from build123d import *

# Parameters (mm, degrees)
F0_R     = 1.5
F0_R_2   = 3.5
F0_R_3   = 1
F0_R_4   = 2.0426148112
F1_DEPTH = 4


with BuildPart() as f1:
    # F0 (on Top) → F1 (new body)
    with BuildSketch(Plane.XY):
        with BuildLine():
            Line((28.2485083335, 43.9163537211), (28.2485083335, 54.5580207216))
            ThreePointArc((28.2485083335, 54.5580207216), (27.1525007025, 57.2380411405), (24.4926270097, 58.38207528))
            Line((24.4926270097, 58.38207528), (15.9756345674, 58.38207528))
            ThreePointArc((15.9756345674, 58.38207528), (11.5015417116, 56.5288453398), (9.6483117715, 52.054752484))
            Line((9.6483117715, 52.054752484), (9.6483117715, 39.0478140861))
            ThreePointArc((9.6483117715, 39.0478140861), (7.7950818313, 34.5737212303), (3.3209889755, 32.7204912901))
            Line((3.3209889755, 32.7204912901), (0, 32.7204912901))
            Line((0, 32.7204912901), (-3.3209889755, 32.7204912901))
            ThreePointArc((-3.3209889755, 32.7204912901), (-7.7950818313, 34.5737212303), (-9.6483117715, 39.0478140861))
            Line((-9.6483117715, 39.0478140861), (-9.6483117715, 52.054752484))
            ThreePointArc((-9.6483117715, 52.054752484), (-11.5015417116, 56.5288453398), (-15.9756345674, 58.38207528))
            Line((-15.9756345674, 58.38207528), (-24.4926270097, 58.38207528))
            ThreePointArc((-24.4926270097, 58.38207528), (-27.1525007025, 57.2380411405), (-28.2485083335, 54.5580207216))
            Line((-28.2485083335, 54.5580207216), (-28.2485083335, 43.9163537211))
            ThreePointArc((-28.2485083335, 43.9163537211), (-30.8923065557, 39.5063295508), (-36.0278336063, 39.759991005))
            Line((-36.0278336063, 39.759991005), (-83.3553595539, 71.4075150422))
            ThreePointArc((-83.3553595539, 71.4075150422), (-83.1773407039, 70.0948228733), (-83.1178410423, 68.7714517117))
            ThreePointArc((-83.1178410423, 68.7714517117), (-86.7609350808, 59.0670533301), (-95.8902072963, 54.1574840073))
            Line((-95.8902072963, 54.1574840073), (-30.0196265199, 1.5012365572))
            ThreePointArc((-30.0196265199, 1.5012365572), (-28.6355347687, -0.2374876701), (-28.1416475773, -2.4042703903))
            Line((-28.1416475773, -2.4042703903), (-28.1416475773, -40))
            ThreePointArc((-28.1416475773, -40), (-28.0556598352, -40.8267401557), (-27.8013775488, -41.6180894438))
            Line((-27.8013775488, -41.6180894438), (-21.7254169173, -55.4257667582))
            ThreePointArc((-21.7254169173, -55.4257667582), (-21.5878462389, -55.7131878969), (-21.4322469923, -55.9912624857))
            Line((-21.4322469923, -55.9912624857), (-10.7166659506, -73.7858242134))
            ThreePointArc((-10.7166659506, -73.7858242134), (-10.1824970033, -75.0266439297), (-10, -76.3651747946))
            Line((-10, -76.3651747946), (-10, -176.3651747946))
            Line((-10, -176.3651747946), (-17.5625588745, -176.3651747946))
            Line((-17.5625588745, -176.3651747946), (-17.5625588745, -183.6033910513))
            Line((-17.5625588745, -183.6033910513), (0, -183.6033910513))
            Line((0, -183.6033910513), (17.5625588745, -183.6033910513))
            Line((17.5625588745, -183.6033910513), (17.5625588745, -176.3651747946))
            Line((17.5625588745, -176.3651747946), (10, -176.3651747946))
            Line((10, -176.3651747946), (10, -76.3651747946))
            ThreePointArc((10, -76.3651747946), (10.1824970033, -75.0266439297), (10.7166659506, -73.7858242134))
            Line((10.7166659506, -73.7858242134), (21.4322469923, -55.9912624857))
            ThreePointArc((21.4322469923, -55.9912624857), (21.5878462389, -55.7131878969), (21.7254169173, -55.4257667582))
            Line((21.7254169173, -55.4257667582), (27.8013775488, -41.6180894438))
            ThreePointArc((27.8013775488, -41.6180894438), (28.0556598352, -40.8267401557), (28.1416475773, -40))
            Line((28.1416475773, -40), (28.1416475773, -2.4042703903))
            ThreePointArc((28.1416475773, -2.4042703903), (28.6355347687, -0.2374876701), (30.0196265199, 1.5012365572))
            Line((30.0196265199, 1.5012365572), (95.8902072963, 54.1574840073))
            ThreePointArc((95.8902072963, 54.1574840073), (85.9348635201, 60.1026484333), (83.3553595539, 71.4075150422))
            Line((83.3553595539, 71.4075150422), (36.0278336063, 39.759991005))
            ThreePointArc((36.0278336063, 39.759991005), (30.8923065557, 39.5063295508), (28.2485083335, 43.9163537211))
        make_face()
        with BuildLine():
            ThreePointArc((0, -96.7485921342), (1.1190603643, -97.1534205019), (1.5911210664, -98.2458218932))
            ThreePointArc((1.5911210664, -98.2458218932), (1.1190603643, -99.3382232845), (0, -99.7430516522))
            ThreePointArc((0, -99.7430516522), (-1.5911210664, -98.2458218932), (0, -96.7485921342))
        make_face(mode=Mode.SUBTRACT)
        with Locations((-15, -44.9954515789)):
            Circle(F0_R, mode=Mode.SUBTRACT)
        with Locations((-66.8339952826, 46.3828593493)):
            Circle(F0_R, mode=Mode.SUBTRACT)
        with Locations((-29.9585536122, 18.5773223639)):
            Circle(F0_R, mode=Mode.SUBTRACT)
        with Locations((-18.9252551645, 47.9994341731)):
            Circle(F0_R, mode=Mode.SUBTRACT)
        with Locations((0, -44.9723601341)):
            Circle(F0_R_2, mode=Mode.SUBTRACT)
        with Locations((15, -44.9954515789)):
            Circle(F0_R, mode=Mode.SUBTRACT)
        with BuildLine():
            ThreePointArc((-10.1997302845, 5.3493127972), (-8.7352641904, 8.8848467031), (-5.1997302845, 10.3493127972))
            Line((-5.1997302845, 10.3493127972), (5.4373050854, 10.3493127972))
            ThreePointArc((5.4373050854, 10.3493127972), (8.9728389913, 8.8848467031), (10.4373050854, 5.3493127972))
            Line((10.4373050854, 5.3493127972), (10.4373050854, -5.1066948846))
            ThreePointArc((10.4373050854, -5.1066948846), (8.9728389913, -8.6422287905), (5.4373050854, -10.1066948846))
            Line((5.4373050854, -10.1066948846), (-5.1997302845, -10.1066948846))
            ThreePointArc((-5.1997302845, -10.1066948846), (-8.7352641904, -8.6422287905), (-10.1997302845, -5.1066948846))
            Line((-10.1997302845, -5.1066948846), (-10.1997302845, 5.3493127972))
        make_face(mode=Mode.SUBTRACT)
        with Locations((18.9252551645, 47.9994341731)):
            Circle(F0_R, mode=Mode.SUBTRACT)
        with Locations((29.9585536122, 18.5773223639)):
            Circle(F0_R, mode=Mode.SUBTRACT)
        with Locations((66.8339952826, 46.3828593493)):
            Circle(F0_R, mode=Mode.SUBTRACT)
        with BuildLine():
            ThreePointArc((112.4534682434, 70.9232873205), (98.1099452114, 83.5161448719), (83.3553595539, 71.4075150422))
            Line((83.3553595539, 71.4075150422), (98.6924420624, 81.6632949003))
            ThreePointArc((98.6924420624, 81.6632949003), (102.2363175022, 82.4481327511), (105.3772742827, 80.6289532416))
            Line((105.3772742827, 80.6289532416), (111.4671739885, 73.0107645192))
            ThreePointArc((111.4671739885, 73.0107645192), (112.0824576726, 72.0247331774), (112.4534682434, 70.9232873205))
        make_face()
        with BuildLine():
            Line((98.6924420624, 81.6632949003), (83.3553595539, 71.4075150422))
            ThreePointArc((83.3553595539, 71.4075150422), (85.9348635201, 60.1026484333), (95.8902072963, 54.1574840073))
            Line((95.8902072963, 54.1574840073), (110.6836880983, 65.9832365143))
            ThreePointArc((110.6836880983, 65.9832365143), (112.0902955562, 67.7694219265), (112.5605632629, 69.9937985024))
            ThreePointArc((112.5605632629, 69.9937985024), (112.514389285, 70.4593924844), (112.4534682434, 70.9232873205))
            ThreePointArc((112.4534682434, 70.9232873205), (112.0824576726, 72.0247331774), (111.4671739885, 73.0107645192))
            Line((111.4671739885, 73.0107645192), (105.3772742827, 80.6289532416))
            ThreePointArc((105.3772742827, 80.6289532416), (102.2363175022, 82.4481327511), (98.6924420624, 81.6632949003))
        make_face()
        with Locations((97.8645756841, 60.7714517117)):
            Circle(F0_R_3, mode=Mode.SUBTRACT)
        with Locations((88.3645756841, 68.7714517117)):
            Circle(F0_R_3, mode=Mode.SUBTRACT)
        with Locations((97.8645756841, 68.7714517117)):
            Circle(F0_R_4, mode=Mode.SUBTRACT)
        with Locations((97.8645756841, 76.7714517117)):
            Circle(F0_R_3, mode=Mode.SUBTRACT)
        with Locations((107.3645756841, 68.7714517117)):
            Circle(F0_R_3, mode=Mode.SUBTRACT)
        with BuildLine():
            ThreePointArc((112.5605632629, 69.9937985024), (112.5288051758, 70.4610534728), (112.4534682434, 70.9232873205))
            ThreePointArc((112.4534682434, 70.9232873205), (112.514389285, 70.4593924844), (112.5605632629, 69.9937985024))
        make_face()
        with BuildLine():
            Line((110.6836880983, 65.9832365143), (95.8902072963, 54.1574840073))
            ThreePointArc((95.8902072963, 54.1574840073), (107.5689740656, 57.6678111084), (112.6113103258, 68.7714517117))
            ThreePointArc((112.6113103258, 68.7714517117), (112.5986180981, 69.3831515852), (112.5605632629, 69.9937985024))
            ThreePointArc((112.5605632629, 69.9937985024), (112.0902955562, 67.7694219265), (110.6836880983, 65.9832365143))
        make_face()
        with BuildLine():
            ThreePointArc((-83.1178410423, 68.7714517117), (-83.1773407039, 70.0948228733), (-83.3553595539, 71.4075150422))
            Line((-83.3553595539, 71.4075150422), (-98.6924420624, 81.6632949003))
            ThreePointArc((-98.6924420624, 81.6632949003), (-102.2363175022, 82.4481327511), (-105.3772742827, 80.6289532416))
            Line((-105.3772742827, 80.6289532416), (-111.4671739885, 73.0107645192))
            ThreePointArc((-111.4671739885, 73.0107645192), (-112.0824576726, 72.0247331774), (-112.4534682434, 70.9232873205))
            ThreePointArc((-112.4534682434, 70.9232873205), (-112.514389285, 70.4593924844), (-112.5605632629, 69.9937985024))
            ThreePointArc((-112.5605632629, 69.9937985024), (-112.0902955562, 67.7694219265), (-110.6836880983, 65.9832365143))
            Line((-110.6836880983, 65.9832365143), (-95.8902072963, 54.1574840073))
            ThreePointArc((-95.8902072963, 54.1574840073), (-86.7609350808, 59.0670533301), (-83.1178410423, 68.7714517117))
        make_face()
        with Locations((-97.8645756841, 60.7714517117)):
            Circle(F0_R_3, mode=Mode.SUBTRACT)
        with Locations((-107.3645756841, 68.7714517117)):
            Circle(F0_R_3, mode=Mode.SUBTRACT)
        with Locations((-97.8645756841, 68.7714517117)):
            Circle(F0_R_4, mode=Mode.SUBTRACT)
        with Locations((-88.3645756841, 68.7714517117)):
            Circle(F0_R_3, mode=Mode.SUBTRACT)
        with Locations((-97.8645756841, 76.7714517117)):
            Circle(F0_R_3, mode=Mode.SUBTRACT)
        with BuildLine():
            Line((-98.6924420624, 81.6632949003), (-83.3553595539, 71.4075150422))
            ThreePointArc((-83.3553595539, 71.4075150422), (-98.1099452114, 83.5161448719), (-112.4534682434, 70.9232873205))
            ThreePointArc((-112.4534682434, 70.9232873205), (-112.0824576726, 72.0247331774), (-111.4671739885, 73.0107645192))
            Line((-111.4671739885, 73.0107645192), (-105.3772742827, 80.6289532416))
            ThreePointArc((-105.3772742827, 80.6289532416), (-102.2363175022, 82.4481327511), (-98.6924420624, 81.6632949003))
        make_face()
        with BuildLine():
            ThreePointArc((-112.5605632629, 69.9937985024), (-112.514389285, 70.4593924844), (-112.4534682434, 70.9232873205))
            ThreePointArc((-112.4534682434, 70.9232873205), (-112.5288051758, 70.4610534728), (-112.5605632629, 69.9937985024))
        make_face()
        with BuildLine():
            ThreePointArc((-112.5605632629, 69.9937985024), (-108.0212046971, 58.0799097421), (-95.8902072963, 54.1574840073))
            Line((-95.8902072963, 54.1574840073), (-110.6836880983, 65.9832365143))
            ThreePointArc((-110.6836880983, 65.9832365143), (-112.0902955562, 67.7694219265), (-112.5605632629, 69.9937985024))
        make_face()
    extrude(amount=F1_DEPTH)


solid = f1.part
Source: CAD feature listing. Evaluate the final solid. Frame: model axes, mm. A direction names the side the tool comes from. Round coordinates to 2 decimals unless told otherwise and drop trailing zeros. Loops run counter-clockwise (first coordinate to the right, second up) from the corner with the lowest first, then second, coordinate; pieces in that order, holes last.
Q1. Ray query, line 1 (Y direction, x = -15, z = 2.4); line 2 (X direction, y = -3, z = 2.55); line 3 (X direction, y = -137, z = 1.55). Return the intervals inside material, ascending.
Q2. Mould query, pull axis X, two halves, no side actions, for faces 1 (the face through (98.4, 83.51, 1.97)), 2 (the face through (-9, -10, 4)), 3 (the face through (24.72, -48.62, 1.97)). Classes: pulls with the +X half, pulls with the -X half, needs draft (parallel to the pull), parting line crosses it, or undercut.
Q3. First-contact query: P1, Ø1.5, axis at y = 51.5, z = 1.5, coming from the -X side; P2, Ø2.5, axis at x = 97.86, y = 68.77, coming from the +Z side; P3, Ø2, axis at y = -27, z = 2.5, coming from the -X side; P4, Ø1, axis at x = -21, z = 2.5, coming from the -Y side. Flat tips, straight axial feed; report the tip coordinate or a pass-through.
Q4. Access query for faces 4 (the face through (16, -65.01, 1.97)), 5 (the face through (-16.15, -64.76, 1.97)), 6 (the face through (-24.806, -48.425, 1.972)), 7 (the face through (11.551, 56.578, 1.972)). Directions: +Z, -Z, +X, -X, +Y, -Y. A direction counts if a zero-diameter tool reaches every point of the face in a straight line with its end or side. Return the directions, or none.
Q5. Section A-A, the plane y = -13. Return loops of the section in (x, z), plus the area to 3 significant figures.
Q6. Section B-B, the plane x = -77.5. Return loops of the section in (y, z).
Q7. Section C-C, the plane z = 0.75. State how many separate pieces and enclosed holes the cut face has, plus the area to 3 significant figures.
Solutions:
1. line 1: y = -183.6 to -176.37, -66.67 to -46.5, -43.5 to 58.31
1. line 2: x = -28.14 to -10.2, 10.44 to 28.14
1. line 3: x = -10 to 10
2. face 1: undercut
2. face 2: needs draft
2. face 3: pulls with the +X half
3. P1: stops at x = -93.5
3. P2: passes through
3. P3: stops at x = -28.14
3. P4: stops at y = -57.54
4. face 4: +Z, -Z, +X
4. face 5: +Z, -Z, -X
4. face 6: +Z, -Z, -X, -Y
4. face 7: +Z, -Z, +Y
5. outline: (-28.14, 0) - (28.14, 0) - (28.14, 4) - (-28.14, 4) - close
5. area: 225 mm2
6. outline: (39.46, 0) - (67.49, 0) - (67.49, 4) - (39.46, 4) - close
7. separate pieces: 1
7. enclosed holes: 21
7. area: 13,200 mm2
